```python
from build123d import *

# Parameters (mm, degrees)
SKETCH1_W           = 60
SKETCH1_H           = 60
BOSS_EXTRUDE1_DEPTH = 50
SKETCH1_4_W         = 60
SKETCH1_4_H         = 60
BOSS_EXTRUDE2_DEPTH = 30
SKETCH3_R           = 15
CUT_EXTRUDE1_DEPTH  = 30
CUT_EXTRUDE3_REACH  = 103.85
CUT_EXTRUDE4_REACH  = 132.508
SKETCH3_3_R         = 15


with BuildPart() as part:
    # Sketch1 → Boss-Extrude1 (new body)
    with BuildSketch(Plane.XY):
        Polygon((-27.961904762, 106.171428571), (-64.628571429, 106.171428571), (-64.628571429, 86.171428571), (-4.628571429, 86.171428571), align=None)
        with Locations((-34.628571429, 56.171428571)):
            Rectangle(SKETCH1_W, SKETCH1_H)
        Polygon((65.371428571, 26.171428571), (-4.628571429, 86.171428571), (-4.628571429, 26.171428571), align=None)
    extrude(amount=-BOSS_EXTRUDE1_DEPTH)

    # Sketch1_4 → Boss-Extrude2 (add)
    with BuildSketch(Plane.XY):
        with Locations((-34.628571429, 56.171428571)):
            Rectangle(SKETCH1_4_W, SKETCH1_4_H)
        Polygon((65.371428571, 26.171428571), (-4.628571429, 86.171428571), (-4.628571429, 26.171428571), align=None)
    extrude(amount=BOSS_EXTRUDE2_DEPTH)

    # Sketch3 → Cut-Extrude1 (cut)
    with BuildSketch(Plane(origin=(40.618487395, 47.388235294, 0), x_dir=(0.7592566023652969, -0.6507913734559682, 0), z_dir=(0.6507913734559682, 0.7592566023652969, 0))):
        with Locations(Location((-33.725710627, 10, 0), (0, 0, 180))):
            Circle(SKETCH3_R)
    extrude(amount=-CUT_EXTRUDE1_DEPTH, mode=Mode.SUBTRACT)

    # Sketch4 → Cut-Extrude3 (cut, up to next)
    with BuildSketch(Plane(origin=(0, 86.171428571, 0), x_dir=(1, 0, 0), z_dir=(0, 1, 0)), mode=Mode.PRIVATE) as cut_extrude3_sk1:
        Polygon((65.371428571, -30), (-4.628571429, -30), (65.371428571, 0), align=None)
    cut_extrude3_tool1 = extrude(cut_extrude3_sk1.sketch, amount=-CUT_EXTRUDE3_REACH, mode=Mode.PRIVATE) & part.part
    add(cut_extrude3_tool1.solids().sort_by_distance((42.038095, 86.171429, 20))[0], mode=Mode.SUBTRACT)

    # Sketch3_3 → Cut-Extrude4 (cut, up to next)
    with BuildSketch(Plane(origin=(40.618487395, 47.388235294, 0), x_dir=(0.7592566023652969, -0.6507913734559682, 0), z_dir=(0.6507913734559682, 0.7592566023652969, 0)), mode=Mode.PRIVATE) as cut_extrude4_sk1:
        with Locations(Location((-33.725710627, 10, 0), (0, 0, 180))):
            Circle(SKETCH3_3_R)
    cut_extrude4_tool1 = extrude(cut_extrude4_sk1.sketch, amount=-CUT_EXTRUDE4_REACH, mode=Mode.PRIVATE) & part.part
    add(cut_extrude4_tool1.solids().sort_by_distance((15.012019, 69.336637, -10))[0], mode=Mode.SUBTRACT)


solid = part.part
```
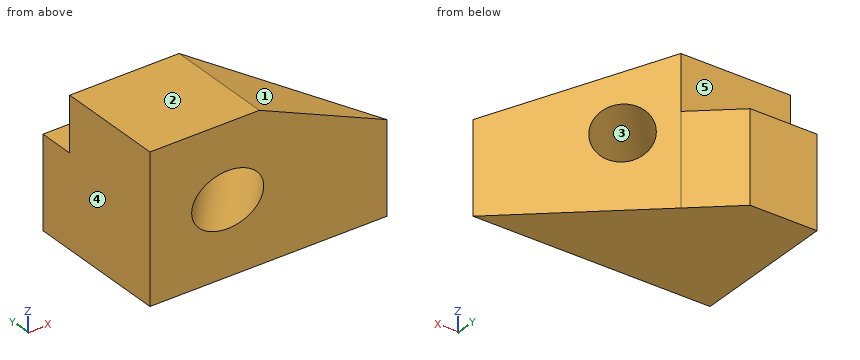
The model under review builds one solid part; all positions refer to its coordinate system, in mm. Face numbers are marked on the shaded views. A direction names the side the tool comes from. Give positions to 0.01 mm unless a question says otherwise; leave off trailing zeros. Write each loop counter-clockwise with the first axis right and the second up, starting at its lowest first coordinate (ties: lowest second). Pieces come first, ordered by that corner, then holes. Notation, with made-up numbers: M -35.5,22 L -6.5,22 A10 ccw -6.5,41 Z; hole C 19,23 d9. An arc over 180 degrees is marked long. Answer in a Markdown table with one row per item.
Item 1: Draft analysis for pull direction X (two halves, no side actions). For the marked faces 1, 2 and 3, state which applies: +X half, -X half, draft (parallel to the pull), parting line (faces both ways), or undercut.
Check sheet entries:
| item | result |
|---|---|
| face 1 | +X half |
| face 2 | draft |
| face 3 | undercut |
Item 2: Add section D-D on z = 17.5. Give the boundary of the cut face in (x, y), plus the area to 3 significant figures.
Check sheet entries:
| item | result |
|---|---|
| outline | M -64.63,26.17 L 24.54,26.17 L 24.54,61.17 L -4.63,86.17 L -64.63,86.17 Z |
| area | 4,990 mm2 |
Item 3: Add section C-C on y = 90. Give the boundary of the cut face in (x, z).
Check sheet entries:
| item | result |
|---|---|
| outline | M -64.63,-50 L -9.1,-50 L -9.1,0 L -64.63,0 Z |
Item 4: For line 1 along Z through (x, y) = (16, 50.5); line 2 along Y through (x, z) = (-23.5, 16); line 3 along X through (y, z) = (50, -18.5), list the stretches that pass through material, from the lowest coordinate up.
Check sheet entries:
| item | result |
|---|---|
| line 1 | -50 to -17.47, -2.53 to 21.16 |
| line 2 | 26.17 to 86.17 |
| line 3 | -64.63 to -17.84, 14.72 to 37.57 |
Item 5: For P1, Ø10, axis at x = -29, y = 98.5, coming from the +Z side; P2, Ø2, axis at x = 39, z = -2, coming from the +Y side; P3, Ø8, axis at x = 23.5, z = -38, coming from the +Y side, all flat-tipped, find the tip position at first contact; note any pin that passes through.
Check sheet entries:
| item | result |
|---|---|
| P1 | z = 0 |
| P2 | y = 49.63 |
| P3 | y = 65.49 |
Item 6: Add section B-B on z = -38. Give the boundary of the cut face in (x, y).
Check sheet entries:
| item | result |
|---|---|
| outline | M -64.63,26.17 L 65.37,26.17 L -27.96,106.17 L -64.63,106.17 Z |
Item 7: Tool access review of the marked faces 4 and 5: name each direction out of +Z, -Z, +X, -X, +Y, -Y from which nothing blocks a thin tool from reaching the whole face with its end or side.
Check sheet entries:
| item | result |
|---|---|
| face 4 | +Z, -Z, -X, +Y, -Y |
| face 5 | +Z, +X, -X, +Y |
Item 8: Add section A-A on x = -48.5. Give the boundary of the cut face in (y, z).
Check sheet entries:
| item | result |
|---|---|
| outline | M 26.17,-50 L 106.17,-50 L 106.17,0 L 86.17,0 L 86.17,30 L 26.17,30 Z |
